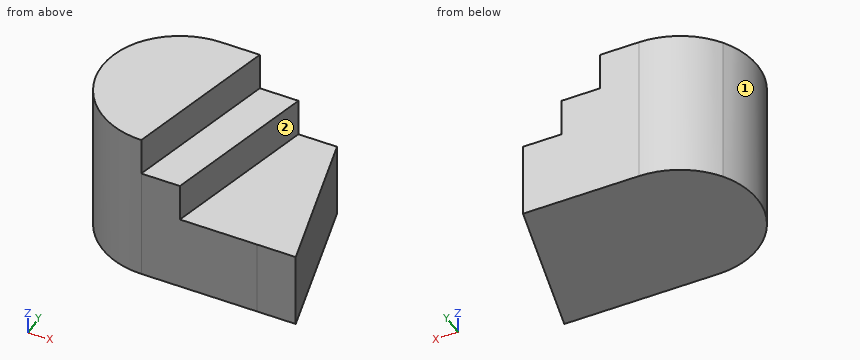
from build123d import *

# Parameters (mm, degrees)
F1_DEPTH = 1016
F3_DEPTH = 254
F6_DEPTH = 508
F7_DEPTH = 25
F8_DEPTH = 100


with BuildPart() as f1:
    # F0 (on Top) → F1 (new body)
    with BuildSketch(Plane.XY):
        with BuildLine():
            Line((762, 513.1272309102), (0, 513.1272309102))
            ThreePointArc((0, 513.1272309102), (-246.0238589032, 453.018466107), (-436.6134349374, 286.2359242663))
            ThreePointArc((-436.6134349374, 286.2359242663), (-522.7640214805, 5.3030259362), (-436.6134349374, -275.629872394))
            ThreePointArc((-436.6134349374, -275.629872394), (-250.137217706, -442.4598438392), (-7.2941860889, -502.7332290138))
            Line((-7.2941860889, -502.7332290138), (754.7058139111, -502.7332290138))
            Line((754.7058139111, -502.7332290138), (1008.7058136281, -502.7452183176))
            Line((1008.7058136281, -502.7452183176), (762, 513.1272309102))
        make_face()
    extrude(amount=F1_DEPTH)

    # F2 (on face) → F3 (cut)
    with BuildSketch(Plane.XY.offset(1016)):
        Polygon((254, 513.1272309102), (-7.2941860889, -502.7332290138), (246.7058139111, -502.7332290138), (508, 513.1272309102), align=None)
    extrude(amount=-F3_DEPTH, mode=Mode.SUBTRACT)

    # F4 (on face) → F6 (cut)
    with BuildSketch(Plane.XY.offset(1016)):
        Polygon((246.7058139111, -502.7332290138), (754.7058139111, -502.7332290138), (1008.7058136281, -502.7452183176), (762, 513.1272309102), (508, 513.1272309102), align=None)
    extrude(amount=-F6_DEPTH, mode=Mode.SUBTRACT)


with BuildPart() as f7:
    # F5 (on face) → F7 (new body)
    with BuildSketch(Plane.XY.offset(1016)):
        Polygon((508, 513.1272309102), (246.7058139111, -502.7332290138), (754.7058139111, -502.7332290138), (1008.7058136281, -502.7452183176), (762, 513.1272309102), align=None)
    extrude(amount=F7_DEPTH)

    # F8 (cut): a face of the model
    f8_faces = [f7.faces().sort_by_distance(p)[0] for p in [
        (630.7450759157, -79.459043637, 1041),
    ]]
    extrude(f8_faces, amount=-F8_DEPTH, mode=Mode.SUBTRACT)


solid = f1.part
Here's how the part is built. I have some questions about the finished solid (model axes, mm). Face numbers are marked on the shaded views. A direction names the side the tool comes from. Coordinates: 2 decimals unless noted, no trailing zeros. Order: outer loops, then holes, each group sorted by start corner. A loop starts at its lowest first (then second) coordinate and runs counter-clockwise, first axis right, second up. Notation, with made-up numbers: M -9.75,-16 L 8.25,-16 A21 cw 8.25,-12 Z; hole C 84.5,5 d7. An arc over 180 degrees is marked long. Answer as CSV lines item,"result". Start each with the question number.
1. I need wall thicknesses on line 1 (Z direction, x = 385, y = -355.5); line 2 (Z direction, x = 116, y = -189); line 3 (Y direction, x = 153.5, z = 261). Which ranges of each line are inside material? Lowest first, please. Write a range as [from, to].
2. I want a section at C-C, the plane x = 640.5. Write out the boundary of the cut face in (y, z).
3. For pin 1 (4 mm diameter, centred on y = -254, z = 402.5, fed in from -X); pin 2 (8 mm diameter, centred on y = 169, z = 595, fed in from -X); pin 3 (10 mm diameter, centred on y = 302.5, z = 884, fed in from +X), each with a flat end and sliding along its axis, tell me the tip position at first contact or that it passes through.
4. On a 3-axis mill with a long thin cutter (end or side, diameter ignored), from which of +Z, -Z, +X, -X, +Y, -Y can I reach the whole of each face in a straight line? I mean the marked faces 1 and 2. Say none if no direction works.
5. I want a section at D-D, the plane z = 895.5. Write out the boundary of the cut face in (x, y).
6. I want a section at B-B, the plane y = 334.5. Write out the boundary of the cut face in (x, z).
7. I want a section at A-A, the plane z = 457.5. Write out the boundary of the cut face in (x, y).
Recorded:
1,line 1,"z = [0, 508]"
1,line 2,"z = [0, 762]"
1,line 3,"y = [-502.73, 513.13]"
2,outline,"M -502.73,0 L 513.13,0 L 513.13,508 L -502.73,508 Z"
3,pin 1,"stops at x = -451.66"
3,pin 2,"stops at x = -496.64"
3,pin 3,"stops at x = 201.11"
4,face 1,"+Z, -Z, -X"
4,face 2,"+Z, +X, -Y"
5,outline,"M -436.61,-275.63 A519.35 ccw -7.29,-502.73 L 254,513.13 L 0,513.13 A533.54 ccw -436.61,286.24 A501.13 ccw Z"
6,outline,"M -398.37,0 L 805.38,0 L 805.38,508 L 462.05,508 L 462.05,762 L 208.05,762 L 208.05,1016 L -398.37,1016 Z"
7,outline,"M -436.61,-275.63 A519.35 ccw -7.29,-502.73 L 754.71,-502.73 L 1008.71,-502.75 L 762,513.13 L 0,513.13 A533.54 ccw -436.61,286.24 A501.13 ccw Z"
